```python
from build123d import *
from OCP.BRepFilletAPI import BRepFilletAPI_MakeChamfer

# Parameters (mm, degrees)
SKETCH_1_W               = 60
SKETCH_1_H               = 20
EXTRUDE_1_DEPTH          = 3
SKETCH_2_W               = 10.25
SKETCH_2_H               = 20
EXTRUDE_2_DEPTH          = 10
CUT_EXTRUDE_1_DEPTH      = 54.113675264
CUT_EXTRUDE_1_DEPTH_BACK = 54.113675264
SKETCH_3_R               = 2
SKETCH_4_R               = 1.4
CUT_EXTRUDE_2_DEPTH      = 54.113675264
EXTRUDE_3_DEPTH          = 10.25
EXTRUDE_4_DEPTH          = 10.25
CUT_EXTRUDE_3_DEPTH      = 3.2
CHAMFER_1_SIZE           = 1.6
CHAMFER_1_SIZE2          = 1.9


with BuildPart() as part:
    # 스케치1 → 보스-돌출1 (new body)
    with BuildSketch(Plane.XY):
        Polygon((-48.25, 18), (48.25, 18), (48.25, 10), (40.25, 10), (40.25, -10), (48.25, -10), (48.25, -18), (-48.25, -18), (-48.25, -10), (-40.25, -10), (-40.25, 10), (-48.25, 10), align=None)
        Rectangle(SKETCH_1_W, SKETCH_1_H, mode=Mode.SUBTRACT)
    extrude(amount=EXTRUDE_1_DEPTH)

    # 스케치2 → 보스-돌출2 (add)
    with BuildSketch(Plane.XY.offset(3)):
        with Locations((35.125, 0)):
            Rectangle(SKETCH_2_W, SKETCH_2_H)
        with Locations((-35.125, 0)):
            Rectangle(SKETCH_2_W, SKETCH_2_H)
    extrude(amount=EXTRUDE_2_DEPTH)

    # 스케치3 → 컷-돌출1 (cut, two sides: drawn at the far end of the back side and taken through both)
    with BuildSketch(Plane(origin=(0, 0, 0), x_dir=(0, 0, -1), z_dir=(1, 0, 0)).offset(-CUT_EXTRUDE_1_DEPTH_BACK)):
        with Locations((-7, 0)):
            Circle(SKETCH_3_R)
    extrude(amount=CUT_EXTRUDE_1_DEPTH + CUT_EXTRUDE_1_DEPTH_BACK, mode=Mode.SUBTRACT)

    # 스케치4 → 컷-돌출2 (cut, through all)
    with BuildSketch(Plane.XY):
        with Locations(Location((44.25, 14, 0), (0, 0, 180))):
            Circle(SKETCH_4_R)
        with Locations(Location((-44.25, 14, 0), (0, 0, 180))):
            Circle(SKETCH_4_R)
        with Locations(Location((44.25, -14, 0), (0, 0, 180))):
            Circle(SKETCH_4_R)
        with Locations(Location((-44.25, -14, 0), (0, 0, 180))):
            Circle(SKETCH_4_R)
    extrude(amount=CUT_EXTRUDE_2_DEPTH, mode=Mode.SUBTRACT)

    # 스케치5 → 보스-돌출3 (add)
    with BuildSketch(Plane(origin=(40.25, 0, 0), x_dir=(0, 0, -1), z_dir=(1, 0, 0))):
        Polygon((-13, 10), (-3, 18), (-3, 10), align=None)
        Polygon((-13, -10), (-3, -10), (-3, -18), align=None)
    extrude(amount=-EXTRUDE_3_DEPTH)

    # 스케치6 → 보스-돌출4 (add)
    with BuildSketch(Plane.ZY.offset(40.25)):
        Polygon((3, 18), (3, 10), (13, 10), align=None)
        Polygon((3, -10), (3, -18), (13, -10), align=None)
    extrude(amount=-EXTRUDE_4_DEPTH)

    # 스케치7 → 컷-돌출3 (cut)
    with BuildSketch(Plane.ZY.offset(-30)):
        Polygon((7, 4.041451884), (3.5, 2.020725942), (3.5, -2.020725942), (7, -4.041451884), (10.5, -2.020725942), (10.5, 2.020725942), align=None)
    cut_extrude_3 = extrude(amount=-CUT_EXTRUDE_3_DEPTH, mode=Mode.SUBTRACT)

    # 대칭 복사2: 컷-돌출3 across plane
    add(cut_extrude_3.mirror(Plane(origin=(0, 0, 0), x_dir=(0, 0, 1), z_dir=(1, 0, 0))), mode=Mode.SUBTRACT)

    # 모따기1: one chamfer whose edges measure the first distance from different faces: ONE call of the kernel's chamfer builder (chamfer() names one face for all edges)
    chamfer_1_edges_1 = [part.edges().sort_by_distance(p)[0] for p in [
        (45.65, -14, 3),
    ]]
    chamfer_1_side_1 = [part.faces().sort_by_distance(p)[0] for p in [
        (44.25, -17.886862915, 3),
    ]]
    chamfer_1_edges_2 = [part.edges().sort_by_distance(p)[0] for p in [
        (-42.85, -14, 3),
    ]]
    chamfer_1_side_2 = [part.faces().sort_by_distance(p)[0] for p in [
        (-44.25, -17.886862915, 3),
    ]]
    chamfer_1_edges_3 = [part.edges().sort_by_distance(p)[0] for p in [
        (45.65, 14, 3),
    ]]
    chamfer_1_side_3 = [part.faces().sort_by_distance(p)[0] for p in [
        (40.363137085, 14, 3),
    ]]
    chamfer_1_edges_4 = [part.edges().sort_by_distance(p)[0] for p in [
        (-42.85, 14, 3),
    ]]
    chamfer_1_side_4 = [part.faces().sort_by_distance(p)[0] for p in [
        (-40.363137085, 14, 3),
    ]]
    chamfer_1 = BRepFilletAPI_MakeChamfer(part.part.solid().wrapped)
    for e in chamfer_1_edges_1:
        chamfer_1.Add(CHAMFER_1_SIZE, CHAMFER_1_SIZE2, e.wrapped, chamfer_1_side_1[0].wrapped)  # the first distance lies on this face
    for e in chamfer_1_edges_2:
        chamfer_1.Add(CHAMFER_1_SIZE, CHAMFER_1_SIZE2, e.wrapped, chamfer_1_side_2[0].wrapped)  # the first distance lies on this face
    for e in chamfer_1_edges_3:
        chamfer_1.Add(CHAMFER_1_SIZE, CHAMFER_1_SIZE2, e.wrapped, chamfer_1_side_3[0].wrapped)  # the first distance lies on this face
    for e in chamfer_1_edges_4:
        chamfer_1.Add(CHAMFER_1_SIZE, CHAMFER_1_SIZE2, e.wrapped, chamfer_1_side_4[0].wrapped)  # the first distance lies on this face
    add(Compound.cast(chamfer_1.Shape()), mode=Mode.REPLACE)


solid = part.part
```
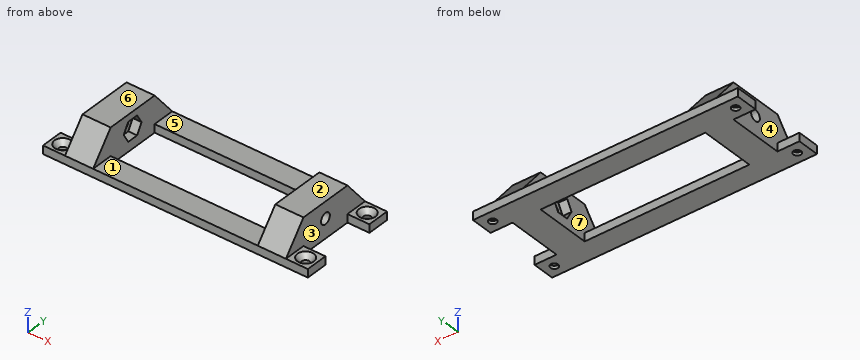
Geometry check sheet. Reference: the model listing, model coordinates, mm. Face numbers are marked on the shaded views. A direction names the side the tool comes from. Round coordinates to 2 decimals unless told otherwise and drop trailing zeros. Loops run counter-clockwise (first coordinate to the right, second up) from the corner with the lowest first, then second, coordinate; pieces in that order, holes last. Notation, with made-up numbers: (81.5, -31) - (111.5, -31) arc R17 ccw to (111.5, -21) - close; hole circle Ø8 at (49, 65.5). An arc over 180 degrees is marked (long way). Use a Markdown table: item, result.
Q1. Cross-section at D-D on z = 8. Record the cut outline in (x, y).
Solutions:
| item | result |
|---|---|
| outline | (-40.25, -14) - (-30, -14) - (-30, -3.46) - (-33.2, -3.46) - (-33.2, -1.73) - (-40.25, -1.73) - close; (-40.25, 1.73) - (-33.2, 1.73) - (-33.2, 3.46) - (-30, 3.46) - (-30, 14) - (-40.25, 14) - close; (30, -14) - (40.25, -14) - (40.25, -1.73) - (33.2, -1.73) - (33.2, -3.46) - (30, -3.46) - close; (30, 3.46) - (33.2, 3.46) - (33.2, 1.73) - (40.25, 1.73) - (40.25, 14) - (30, 14) - close |
Q2. Access from +Z, -Z, +X, -X, +Y, -Y to the whole of each face (thin tool, end or side, straight path). Record for the marked faces 5, 6 and 7.
Solutions:
| item | result |
|---|---|
| face 5 | +Z, +Y, -Y |
| face 6 | +Z, +X, -X, +Y, -Y |
| face 7 | +Z |
Q3. Draft check along X on the marked faces 1, 2, 3 and 4. Enter one of: released by +X, released by -X, zero draft, split by the parting line, or undercut.
Solutions:
| item | result |
|---|---|
| face 1 | undercut |
| face 2 | zero draft |
| face 3 | released by +X |
| face 4 | released by -X |
Q4. Go/stop test with flat-tipped pins: P1, Ø1, axis at x = -15.5, y = 9, coming from the +Z side; P2, Ø2, axis at y = -1, z = 7.5, coming from the +X side; P3, Ø2.5, axis at x = -45, y = -13, coming from the +Z side; P4, Ø7.5, axis at y = 2, z = 8, coming from the -X side. Record where each tip stops, or that it passes through.
Solutions:
| item | result |
|---|---|
| P1 | passes through |
| P2 | stops at x = 40.25 |
| P3 | stops at z = 2.41 |
| P4 | stops at x = -40.25 |
Q5. Cross-section at A-A on y = 14. Record the cut outline in (x, z), plus the area to 3 significant figures.
Solutions:
| item | result |
|---|---|
| outline | (-48.25, 0) - (-45.65, 0) - (-45.65, 1.1) - (-47.25, 3) - (-48.25, 3) - close; (-42.85, 0) - (42.85, 0) - (42.85, 1.1) - (41.25, 3) - (40.25, 3) - (40.25, 8) - (30, 8) - (30, 3) - (-30, 3) - (-30, 8) - (-40.25, 8) - (-40.25, 3) - (-41.25, 3) - (-42.85, 1.1) - close; (45.65, 0) - (48.25, 0) - (48.25, 3) - (47.25, 3) - (45.65, 1.1) - close |
| area | 369 mm2 |
Q6. Cross-section at C-C on y = 0. Record the cut outline in (x, z), plus the area to 3 significant figures.
Solutions:
| item | result |
|---|---|
| outline | (-40.25, 0) - (-30, 0) - (-30, 3.5) - (-33.2, 3.5) - (-33.2, 5) - (-40.25, 5) - close; (-40.25, 9) - (-33.2, 9) - (-33.2, 10.5) - (-30, 10.5) - (-30, 13) - (-40.25, 13) - close; (30, 0) - (40.25, 0) - (40.25, 5) - (33.2, 5) - (33.2, 3.5) - (30, 3.5) - close; (30, 10.5) - (33.2, 10.5) - (33.2, 9) - (40.25, 9) - (40.25, 13) - (30, 13) - close |
| area | 165 mm2 |
Q7. Material ranges on line 1 (Y direction, x = -44.25, z = 0.55); line 2 (X direction, y = 14, z = 0.35); line 3 (X direction, y = -8, z = 10), recorded low to high.
Solutions:
| item | result |
|---|---|
| line 1 | y = -18 to -15.4, -12.6 to -10, 10 to 12.6, 15.4 to 18 |
| line 2 | x = -48.25 to -45.65, -42.85 to 42.85, 45.65 to 48.25 |
| line 3 | x = -40.25 to -30, 30 to 40.25 |
Q8. Cross-section at B-B on x = 3. Record the cut outline in (y, z), plus the area to 3 significant figures.
Solutions:
| item | result |
|---|---|
| outline | (-18, 0) - (-10, 0) - (-10, 3) - (-18, 3) - close; (10, 0) - (18, 0) - (18, 3) - (10, 3) - close |
| area | 48.0 mm2 |
